For this review, use the dimensioned drawing (mm, ordinates from the lowest corner) and the shaded views. A direction names the side the tool comes from. Coordinates: 2 decimals unless noted, no trailing zeros. Loops run counter-clockwise (first coordinate to the right, second up) from the corner with the lowest first, then second, coordinate; pieces in that order, holes last. Notation, with made-up numbers: (87, -5.75) - (125, -5.75) arc R9 ccw to (125, 4.25) - close; hole circle Ø3 at (35.5, 21.25). An arc over 180 degrees is marked (long way). Use one line per item in the form item = value. Start each with the question number.
(1) Add section D-D (z = 12.25). State the section outline as (x, y) points, plus the area to 3 significant figures.
(2) Add section C-C (x = 23). State the section outline as (y, z) points.
(3) Clearance check with flat-ended pins moving along their axes: pin 1 Ø8 at (x, y) = (15.5, 16) entering from +Z; pin 2 Ø6 at (x, z) = (27.5, 13.5) entering from +Y; pin 3 Ø1 at (y, z) = (5.5, 20) entering from -X; pin 4 Ø8 at (x, y) = (6, 8) entering from +Z (3 decimals). State where each tip first meets the part, or that it passes through.
(4) Tool access review of the marked faces 4, 5 and 6: name each direction out of +Z, -Z, +X, -X, +Y, -Y from which nothing blocks a thin tool from reaching the whole face with its end or side.
(5) Add section B-B (y = 12.25). State the section outline as (x, z) points, plus the area to 3 significant figures.
(6) For L1, parallel to Z at x = 25, y = 17.5; L2, parallel to X at y = 8.5, z = 5.5; L3, parallel to X at y = 3.5, z = 16.75, list the stretches that pass through material, from the lowest coordinate up.
(7) The part is to be moulded in two halves that separate along Z. For the marked faces 1, 2 and 3, say which applies: pulls with the +Z half, pulls with the -Z half, needs draft (parallel to the pull), parting line crosses it, or undercut.
(8) Add section A-A (z = 24.25). State the section outline as (x, y) points.
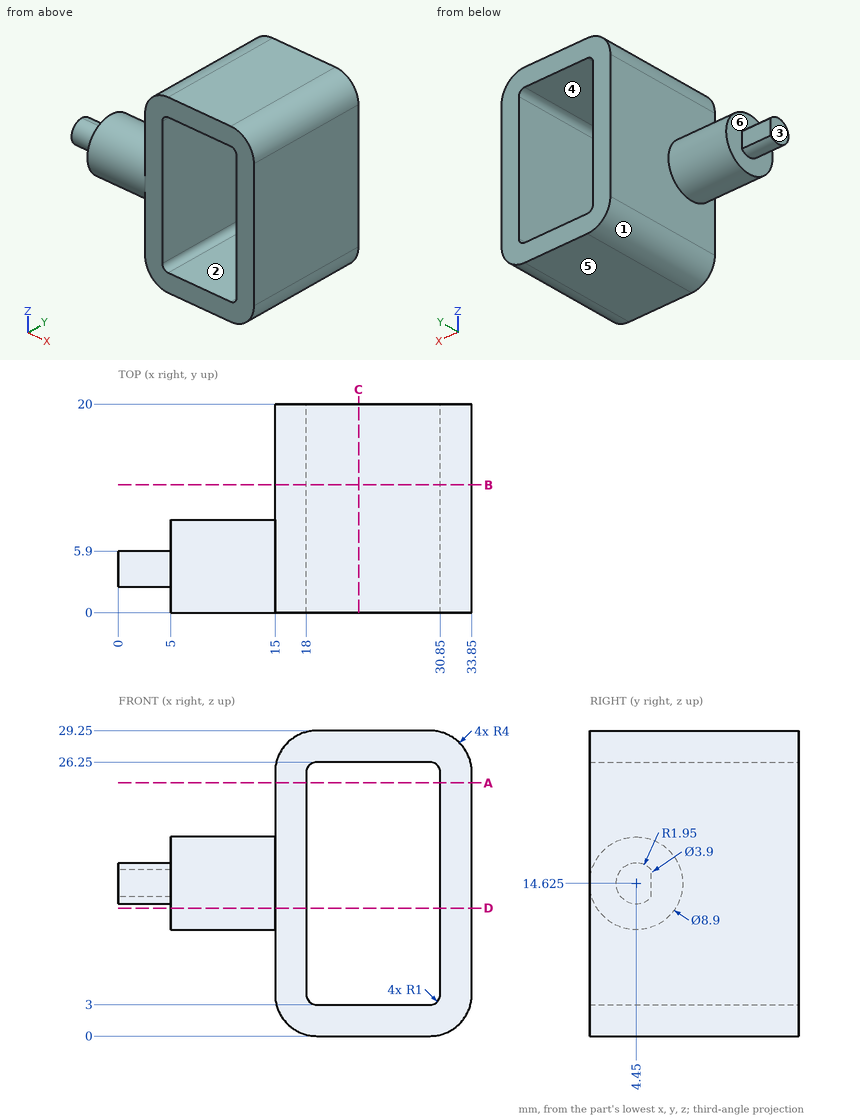
Computed values:
q1.outline = (5, 0.69) - (15, 0.69) - (15, 0) - (18, 0) - (18, 20) - (15, 20) - (15, 8.21) - (5, 8.21) - close; (30.85, 0) - (33.85, 0) - (33.85, 20) - (30.85, 20) - close
q1.area = 195 mm^2
q2.outline = (0, 0) - (20, 0) - (20, 3) - (0, 3) - close; (0, 26.25) - (20, 26.25) - (20, 29.25) - (0, 29.25) - close
q3.pin_1 = 29.25
q3.pin_2 = through
q3.pin_3 = 15
q3.pin_4 = 19.075
q4.face_4 = +Y, -Y
q4.face_5 = -Z, +X, -X, +Y, -Y
q4.face_6 = -X
q5.outline = (15, 4) arc R4 ccw to (19, 0) - (29.85, 0) arc R4 ccw to (33.85, 4) - (33.85, 25.25) arc R4 ccw to (29.85, 29.25) - (19, 29.25) arc R4 ccw to (15, 25.25) - close; hole (18, 4) arc R1 ccw to (19, 3) - (29.85, 3) arc R1 ccw to (30.85, 4) - (30.85, 25.25) arc R1 ccw to (29.85, 26.25) - (19, 26.25) arc R1 ccw to (18, 25.25) - close
q5.area = 240 mm^2
q6.L1 = 0 to 3, 26.25 to 29.25
q6.L2 = 15 to 18, 30.85 to 33.85
q6.L3 = 5 to 18, 30.85 to 33.85
q7.face_1 = pulls with the -Z half
q7.face_2 = undercut
q7.face_3 = needs draft
q8.outline = (15, 0) - (18, 0) - (18, 20) - (15, 20) - close; (30.85, 0) - (33.85, 0) - (33.85, 20) - (30.85, 20) - close
